```python
from build123d import *

# Parameters (mm, degrees)
BASPROSKE_W         = 10
BASPROSKE_H         = 13.75
TOOTHCUT_DEPTH      = 22.866069606
TEETHCUTS_COUNT     = 20
TEETHCUTS_ANGLE     = 342
BORSKE_R            = 2
BORE_DEPTH          = 50.0000508
SKETCH2_R           = 2
BOSS_EXTRUDE1_DEPTH = 10
SKETCH3_R           = 3.4
BOSS_EXTRUDE2_DEPTH = 6


with BuildPart() as part:
    # BasProSke → Base-Revolve (revolve)
    with BuildSketch(Plane(origin=(0, 0, 0), x_dir=(1, 0, 0), z_dir=(0, 1, 0)), mode=Mode.PRIVATE) as base_revolve_sk:
        with Locations((5, 6.875)):
            Rectangle(BASPROSKE_W, BASPROSKE_H)
    revolve(base_revolve_sk.sketch.rotate(Axis((-10, 0, 0), (1, 0, 0)), 180), axis=Axis((-10, 0, 0), (1, 0, 0)))

    # TooCutSke → ToothCut (cut, through all)
    with BuildSketch(Plane(origin=(0, 0, 0), x_dir=(0, 0, -1), z_dir=(1, 0, 0))):
        with BuildLine():
            ThreePointArc((0.62110296, 10.918848994), (0, 10.9365), (-0.62110296, 10.918848994))
            ThreePointArc((-0.62110296, 10.918848994), (-1.024517052, 12.378857135), (-1.846615859, 13.651067908))
            ThreePointArc((-1.846615859, 13.651067908), (0, 13.7754), (1.846615859, 13.651067908))
            ThreePointArc((1.846615859, 13.651067908), (1.024517052, 12.378857135), (0.62110296, 10.918848994))
        make_face()
    toothcut = extrude(amount=TOOTHCUT_DEPTH, mode=Mode.SUBTRACT)

    # TeethCuts: ToothCut ×20 about axis
    teethcuts_axis = Axis((-10, 0, 0), (1, 0, 0))
    for i in range(1, TEETHCUTS_COUNT):
        add(toothcut.rotate(teethcuts_axis, i * TEETHCUTS_ANGLE / (TEETHCUTS_COUNT - 1)), mode=Mode.SUBTRACT)

    # BorSke → Bore (cut, symmetric)
    with BuildSketch(Plane(origin=(0, 0, 0), x_dir=(0, 0, -1), z_dir=(1, 0, 0))):
        with Locations(Location((0, 0, 0), (0, 0, 180))):
            Circle(BORSKE_R)
    extrude(amount=BORE_DEPTH, both=True, mode=Mode.SUBTRACT)

    # Sketch2 → Boss-Extrude1 (add)
    with BuildSketch(Plane(origin=(10, 0, 0), x_dir=(0, 0, -1), z_dir=(1, 0, 0))):
        Circle(SKETCH2_R)
    extrude(amount=-BOSS_EXTRUDE1_DEPTH)

    # Sketch3 → Boss-Extrude2 (add)
    with BuildSketch(Plane(origin=(10, 0, 0), x_dir=(0, 0, -1), z_dir=(1, 0, 0))):
        with Locations(Location((0, 0, 0), (0, 0, 180))):
            Circle(SKETCH3_R)
    extrude(amount=BOSS_EXTRUDE2_DEPTH)


solid = part.part
```
Check sheet for the modelled part. Datum: model origin and axes. Units: mm. A direction names the side the tool comes from. Round coordinates to 2 decimals unless told otherwise and drop trailing zeros. Order: outer loops, then holes, each group sorted by start corner. A loop starts at its lowest first (then second) coordinate and runs counter-clockwise, first axis right, second up. Notation, with made-up numbers: (48, 12) - (92, 12) arc R19 ccw to (92, 25) - close; hole circle Ø9 at (70.25, 47.5). An arc over 180 degrees is marked (long way). Write item = value, one per line.
Q1. Go/stop test with flat-tipped pins: pin 1 (5 mm diameter, centred on y = 8, z = -1, fed in from -X); pin 2 (5 mm diameter, centred on x = 6.5, z = 3.5, fed in from -Y); pin 3 (6 mm diameter, centred on x = 5.5, y = -8.5, fed in from +Z); pin 4 (1.5 mm diameter, centred on y = 10, z = -4.5, fed in from +X). Record where each tip stops, or that it passes through.
Computed:
pin_1 = 0
pin_2 = -13.63
pin_3 = 12.4
pin_4 = 10
Q2. Draft check along Z on faces 1 (the face through (12.96, 3.32, -0.74)), 2 (the face through (4.93, 12.35, 1.01)), 3 (the face through (10, -3, -3)). Enter one of: pulls with the +Z half, pulls with the -Z half, needs draft (parallel to the pull), parting line crosses it, or undercut.
Computed:
face_1 = parting line crosses it
face_2 = undercut
face_3 = needs draft
Q3. Section check D-D (z = -5). Record the boundary of the cut face in (x, y), and give its area (3 significant figures).
Computed:
outline = (0, -11.67) - (10, -11.67) - (10, 11.67) - (0, 11.67) - close
area = 233 mm^2
Q4. Section check C-C (x = 11.25). Record the boundary of the cut face in (y, z), and give its area (3 significant figures).
Computed:
outline = circle Ø6.8 at (0, 0)
area = 36.3 mm^2
Q5. Section check A-A (y = 0). Record the boundary of the cut face in (x, z), and give its area (3 significant figures).
Computed:
outline = (0, -10.94) - (10, -10.94) - (10, -3.4) - (16, -3.4) - (16, 3.4) - (10, 3.4) - (10, 10.94) - (0, 10.94) - close
area = 260 mm^2
Q6. Tool access check on faces 4 (the face through (4.93, -12.35, -1.01)), 5 (the face through (4.93, 11.461, -4.804)), 6 (the face through (4.93, 1.027, 12.384)), 7 (the face through (4.93, -10.58, 6.44)), 8 (the face through (4.93, -4.804, -11.461)). Record the directions out of +Z, -Z, +X, -X, +Y, -Y that give a thin tool (end or side, any length) a straight path to the whole face; none if there is none.
Computed:
face_4 = +X, -X, -Y
face_5 = +X, -X, +Y
face_6 = +Z, +X, -X
face_7 = +X, -X
face_8 = -Z, +X, -X
Q7. Thickness scan on line 1 along Y through (x, z) = (7.25, 11.5); line 2 along Z through (x, y) = (1.5, -11.75); line 3 along Y through (x, z) = (6, 9). Record the ranges inside material, lowest first.
Computed:
line_1 = -6.55 to -4.84, -2.88 to -0.72, 0.72 to 2.88, 4.84 to 6.55
line_2 = -6.55 to -5.09, -2.88 to -0.79, 0.79 to 2.88, 5.09 to 6.55
line_3 = -9.81 to -7.49, -6.21 to 6.21, 7.49 to 9.81
